Source: CAD feature listing. Evaluate the final solid. Frame: model axes, mm. Face numbers are marked on the shaded views. A direction names the side the tool comes from. Give positions to 0.01 mm unless a question says otherwise; leave off trailing zeros. Loops run counter-clockwise (first coordinate to the right, second up) from the corner with the lowest first, then second, coordinate; pieces in that order, holes last. Notation, with made-up numbers: M 5,-37 L 29,-37 A14 ccw 29,-28 Z; hole C 50,3 d1. An arc over 180 degrees is marked long. Answer in a Markdown table with one row per item.
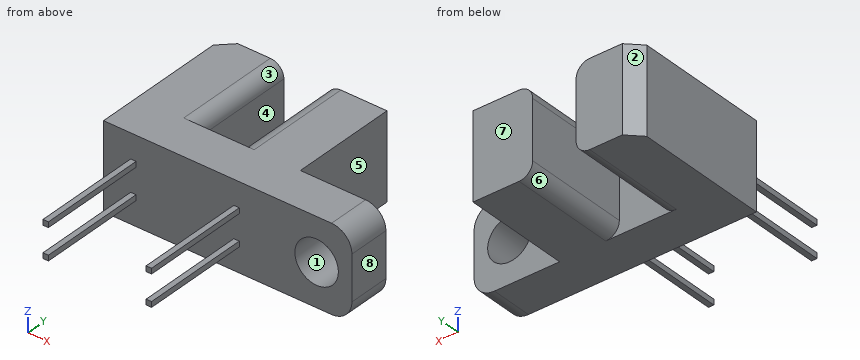
```python
from build123d import *

# Parameters (mm, degrees)
SKETCH1_W                  = 18.3
SKETCH1_H                  = 6.3
BOSS_EXTRUDE1_DEPTH        = 3.1
FILLET1_R                  = 1.5
SKETCH2_W                  = 12
SKETCH2_H                  = 6.3
BOSS_EXTRUDE2_DEPTH        = 7.9
F_3_2_3_2_DIAMETER_HOLE1_D = 3.2
SKETCH5_W                  = 3.2
SKETCH5_H                  = 7.9
CUT_EXTRUDE1_DEPTH         = 16.633697579
CHAMFER1_SIZE              = 1
FILLET2_R                  = 1
SKETCH6_W                  = 0.4
SKETCH6_H                  = 0.4
BOSS_EXTRUDE3_DEPTH        = 8
LPATTERN1_COUNT            = 2
LPATTERN1_PITCH            = 7.6


with BuildPart() as part:
    # Sketch1 → Boss-Extrude1 (new body)
    with BuildSketch(Plane(origin=(0, 0, 0), x_dir=(1, 0, 0), z_dir=(0, 1, 0))):
        Rectangle(SKETCH1_W, SKETCH1_H)
    extrude(amount=BOSS_EXTRUDE1_DEPTH)

    # Fillet1
    fillet1_edges = [part.edges().sort_by_distance(p)[0] for p in [
        (9.15, 1.55, 3.15),
        (9.15, 1.55, -3.15),
    ]]
    fillet(fillet1_edges, radius=FILLET1_R)

    # Sketch2 → Boss-Extrude2 (add)
    with BuildSketch(Plane(origin=(0, 3.1, 0), x_dir=(1, 0, 0), z_dir=(0, 1, 0))):
        with Locations((-3.15, 0)):
            Rectangle(SKETCH2_W, SKETCH2_H)
    extrude(amount=BOSS_EXTRUDE2_DEPTH)

    # Ø3.2 (3.2) Diameter Hole1 (through all)
    with Locations(Plane(origin=(0, 3.1, 0), x_dir=(1, 0, 0), z_dir=(0, 1, 0))):
        with Locations((6.55, 0)):
            Hole(F_3_2_3_2_DIAMETER_HOLE1_D / 2)

    # Sketch5 → Cut-Extrude1 (cut, through all)
    with BuildSketch(Plane.XY.offset(3.15)):
        with Locations((-3.15, 7.05)):
            Rectangle(SKETCH5_W, SKETCH5_H)
    extrude(amount=-CUT_EXTRUDE1_DEPTH, mode=Mode.SUBTRACT)

    # Chamfer1
    chamfer1_edges = [part.edges().sort_by_distance(p)[0] for p in [
        (-9.15, 11, 0),
    ]]
    chamfer(chamfer1_edges, length=CHAMFER1_SIZE)

    # Fillet2
    fillet2_edges = [part.edges().sort_by_distance(p)[0] for p in [
        (-4.75, 7.05, -3.15),
        (-1.55, 7.05, -3.15),
        (-4.75, 7.05, 3.15),
        (-1.55, 7.05, 3.15),
    ]]
    fillet(fillet2_edges, radius=FILLET2_R)

    # Sketch6 → Boss-Extrude3 (add)
    with BuildSketch(Plane.XZ):
        with Locations((0.65, 1.15)):
            Rectangle(SKETCH6_W, SKETCH6_H)
        with Locations((0.65, -1.15)):
            Rectangle(SKETCH6_W, SKETCH6_H)
    boss_extrude3 = extrude(amount=BOSS_EXTRUDE3_DEPTH)

    # LPattern1: Boss-Extrude3 ×2
    with Locations(*[(-i * LPATTERN1_PITCH, 0, 0) for i in range(1, LPATTERN1_COUNT)]):
        add(boss_extrude3)


solid = part.part
```
Q1. Section query C-C (x = 6.55). Output: boundary loops of the cut face in (y, z).
Values follow:
| item | result |
|---|---|
| outline | M 0,-3.15 L 3.1,-3.15 L 3.1,-1.6 L 0,-1.6 Z; M 0,1.6 L 3.1,1.6 L 3.1,3.15 L 0,3.15 Z |
Q2. Contact query for flat-ended pins moving along their axis: pin 1 Ø3 at (x, z) = (7, 1) entering from +Y; pin 2 Ø3 at (y, z) = (5, -2) entering from +X; pin 3 Ø1.9 at (x, z) = (-1, 0) entering from -Y. Output: stop coordinate, or through.
Values follow:
| item | result |
|---|---|
| pin 1 | y = 3.1 |
| pin 2 | x = 2.85 |
| pin 3 | y = 0 |
Q3. Ray query, probe 1 along Z at (x, y) = (6.55, 1.2); probe 2 along Z at (x, y) = (-7, -0.25); probe 3 along Y at (x, z) = (3.75, 2.5). Return the intervals inside material, ascending. Write a range as from..to.
Values follow:
| item | result |
|---|---|
| probe 1 | -3.15..-1.6, 1.6..3.15 |
| probe 2 | -1.35..-0.95, 0.95..1.35 |
| probe 3 | 0..3.1 |
Q4. Reachability of the marked faces 4, 5, 6, 7 and 8 from +Z, -Z, +X, -X, +Y, -Y: full face, straight path, thin tool, end or side. Return the list, or none.
Values follow:
| item | result |
|---|---|
| face 4 | +Z, -Z, +Y |
| face 5 | +Z, -Z, +X, +Y |
| face 6 | -Z, +Y |
| face 7 | +Z, -Z, +X, -X, +Y |
| face 8 | +Z, -Z, +X, +Y, -Y |
Q5. Mould query, pull axis Z, two halves, no side actions, for the marked faces 1, 2 and 3. Classes: +Z half, -Z half, draft (parallel to the pull), parting line (faces both ways), or undercut.
Values follow:
| item | result |
|---|---|
| face 1 | undercut |
| face 2 | draft |
| face 3 | +Z half |
Q6. Section query B-B (z = 0). Output: boundary loops of the cut face in (x, y).
Values follow:
| item | result |
|---|---|
| outline | M -9.15,0 L 4.95,0 L 4.95,3.1 L 2.85,3.1 L 2.85,11 L -1.55,11 L -1.55,3.1 L -4.75,3.1 L -4.75,11 L -8.15,11 L -9.15,10 Z; M 8.15,0 L 9.15,0 L 9.15,3.1 L 8.15,3.1 Z |
Q7. Section query A-A (y = 4.75). Output: boundary loops of the cut face in (x, z), plus the area to 3 significant figures.
Values follow:
| item | result |
|---|---|
| outline | M -9.15,-3.15 L -5.75,-3.15 A1 ccw -4.75,-2.15 L -4.75,2.15 A1 ccw -5.75,3.15 L -9.15,3.15 Z; M -1.55,-2.15 A1 ccw -0.55,-3.15 L 2.85,-3.15 L 2.85,3.15 L -0.55,3.15 A1 ccw -1.55,2.15 Z |
| area | 54.6 mm^2 |
Q8. Section query D-D (y = -1.5). Output: boundary loops of the cut face in (x, z).
Values follow:
| item | result |
|---|---|
| outline | M -7.15,-1.35 L -6.75,-1.35 L -6.75,-0.95 L -7.15,-0.95 Z; M -7.15,0.95 L -6.75,0.95 L -6.75,1.35 L -7.15,1.35 Z; M 0.45,-1.35 L 0.85,-1.35 L 0.85,-0.95 L 0.45,-0.95 Z; M 0.45,0.95 L 0.85,0.95 L 0.85,1.35 L 0.45,1.35 Z |
